```python
from build123d import *

# Parameters (mm, degrees)
SKETCH1_W           = 177.8
SKETCH1_H           = 177.8
BOSS_EXTRUDE1_DEPTH = 15
SKETCH2_W           = 158.75
SKETCH2_H           = 158.75
CUT_EXTRUDE1_DEPTH  = 10
FILLET1_R           = 10
SKETCH3_W           = 63.5
SKETCH3_H           = 63.5
BOSS_EXTRUDE2_DEPTH = 10


with BuildPart() as part:
    # Sketch1 → Boss-Extrude1 (new body)
    with BuildSketch(Plane.XY):
        with Locations((97.785967035, 49.382663919)):
            Rectangle(SKETCH1_W, SKETCH1_H)
    extrude(amount=BOSS_EXTRUDE1_DEPTH)

    # Sketch2 → Cut-Extrude1 (cut)
    with BuildSketch(Plane.XY.offset(15)):
        with Locations((97.785967035, 49.382663919)):
            Rectangle(SKETCH2_W, SKETCH2_H)
    extrude(amount=-CUT_EXTRUDE1_DEPTH, mode=Mode.SUBTRACT)

    # Fillet1
    fillet1_edges = [part.edges().sort_by_distance(p)[0] for p in [
        (177.160967035, 128.757663919, 10),
        (177.160967035, -29.992336081, 10),
        (18.410967035, -29.992336081, 10),
        (18.410967035, 128.757663919, 10),
        (8.885967035, 138.282663919, 7.5),
        (186.685967035, 138.282663919, 7.5),
        (186.685967035, -39.517336081, 7.5),
        (8.885967035, -39.517336081, 7.5),
    ]]
    fillet(fillet1_edges, radius=FILLET1_R)

    # Sketch3 → Boss-Extrude2 (add)
    with BuildSketch(Plane(origin=(0, 0, 0), x_dir=(-1, 0, 0), z_dir=(0, 0, -1))):
        with Locations((-97.785967035, 49.382663919)):
            Rectangle(SKETCH3_W, SKETCH3_H)
    extrude(amount=BOSS_EXTRUDE2_DEPTH)


solid = part.part
```
Verification items for the finished model (mm, model axes). A direction names the side the tool comes from. Give positions to 0.01 mm unless a question says otherwise; leave off trailing zeros. Order: outer loops, then holes, each group sorted by start corner. A loop starts at its lowest first (then second) coordinate and runs counter-clockwise, first axis right, second up. Notation, with made-up numbers: (53.25, 81.25) - (60.25, 81.25) arc R16 ccw to (60.25, 89.25) - close; hole circle Ø11 at (5.25, 79.25). An arc over 180 degrees is marked (long way). Answer as CSV lines item,"result". Start each with the question number.
Item 1: Section check D-D, the plane z = -5.5. Record the boundary of the cut face in (x, y), plus the area to 3 significant figures.
Item 2: Gauge pin test, flat ends, axial feed: pin 1 (4 mm diameter, centred on x = 166, y = 101, fed in from -Z); pin 2 (4 mm diameter, centred on x = 81.5, y = 16.5, fed in from +Z); pin 3 (3 mm diameter, centred on y = 39.5, z = -2.5, fed in from -X). Record the tip position at first contact, or that the pin passes through.
Item 3: Material ranges on L1, parallel to X at y = 39.5, z = 7.75; L2, parallel to Y at x = 127, z = 8.5; L3, parallel to Z at x = 176, y = 87, recorded low to high.
Item 4: Section check C-C, the plane x = 93. Record the boundary of the cut face in (y, z).
Item 5: Section check A-A, the plane z = 11. Record the boundary of the cut face in (x, y), plus the area to 3 significant figures.
Item 6: Section check B-B, the plane y = 46. Record the boundary of the cut face in (x, z).
Item 7: Access from +Z, -Z, +X, -X, +Y, -Y to the whole of each face (thin tool, end or side, straight path). Record for faces 1 (the face through (97, 50, 5)), 2 (the face through (98, 17.633, -5)), 3 (the face through (98, 81.133, -5)), 4 (the face through (129.536, 49, -5)).
Item 8: Mould release check, pull along X, two halves, no side actions. Record for faces 5 (the face through (183.679, -36.666, 7.605)), 6 (the face through (18.411, 48, 10)), 7 (the face through (11.74, 135.28, 7.6)): released by +X, released by -X, zero draft, split by the parting line, or undercut.
Filled in:
1,outline,"(66.04, 17.63) - (129.54, 17.63) - (129.54, 81.13) - (66.04, 81.13) - close"
1,area,"4,030 mm^2"
2,pin 1,"z = 0"
2,pin 2,"z = 5"
2,pin 3,"x = 66.04"
3,L1,"8.89 to 18.41, 177.16 to 186.69"
3,L2,"-39.52 to -29.99, 128.76 to 138.28"
3,L3,"0 to 5"
4,outline,"(-39.52, 0) - (17.63, 0) - (17.63, -10) - (81.13, -10) - (81.13, 0) - (138.28, 0) - (138.28, 15) - (128.76, 15) - (128.76, 5) - (-29.99, 5) - (-29.99, 15) - (-39.52, 15) - close"
5,outline,"(8.89, -29.52) arc R10 ccw to (18.89, -39.52) - (176.69, -39.52) arc R10 ccw to (186.69, -29.52) - (186.69, 128.28) arc R10 ccw to (176.69, 138.28) - (18.89, 138.28) arc R10 ccw to (8.89, 128.28) - close; hole (18.41, -19.99) arc R10 ccw to (28.41, -29.99) - (167.16, -29.99) arc R10 ccw to (177.16, -19.99) - (177.16, 118.76) arc R10 ccw to (167.16, 128.76) - (28.41, 128.76) arc R10 ccw to (18.41, 118.76) - close"
5,area,"6,410 mm^2"
6,outline,"(8.89, 0) - (66.04, 0) - (66.04, -10) - (129.54, -10) - (129.54, 0) - (186.69, 0) - (186.69, 15) - (177.16, 15) - (177.16, 5) - (18.41, 5) - (18.41, 15) - (8.89, 15) - close"
7,face 1,"+Z"
7,face 2,"-Z, +X, -X, -Y"
7,face 3,"-Z, +X, -X, +Y"
7,face 4,"-Z, +X, +Y, -Y"
8,face 5,"released by +X"
8,face 6,"undercut"
8,face 7,"released by -X"
